The drawing under review shows one solid part. Ordinate dimensions are in mm from its lowest x, y, z. Round coordinates to 2 decimals unless told otherwise and drop trailing zeros. Write each loop counter-clockwise with the first axis right and the second up, starting at its lowest first coordinate (ties: lowest second). Pieces come first, ordered by that corner, then holes. Notation, with made-up numbers: (-15, 44) - (23, 44) arc R12 cw to (23, 60) - close; hole circle Ø11 at (-29.75, 42). An arc over 180 degrees is marked (long way). Answer in a Markdown table with one row per item. Add a question column.
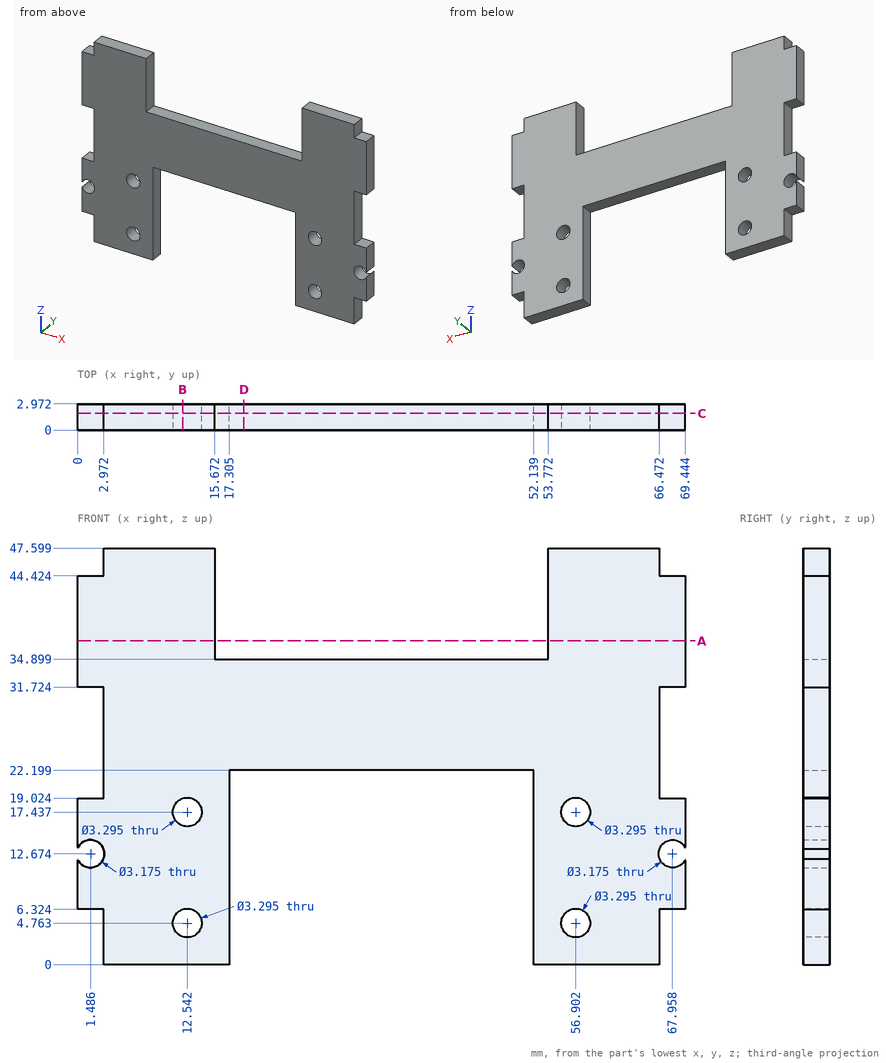
Q1. Add section A-A on z = 37. State the section outline as (x, y) points.
Q2. To check wall thickness, follow probe 1 along X at (y, z) = (2.55, 46); probe 2 along Z at (x, y) = (57, 2.55); probe 3 along Z at (x, y) = (56.5, 2) (1 decimal). State the ranges of each line that lie inside material, in increasing order.
Q3. Add section D-D on x = 19. State the section outline as (y, z) points.
Q4. Add section B-B on x = 12. State the section outline as (y, z) points, then the cut area to 3 significant figures.
Q5. Insertion check: pin 1 Ø0.9 at (x, y) = (67.5, 2) entering from +Z; pin 2 Ø0.9 at (x, y) = (1, 2) entering from -Z. Each pin has a flat end and moves straight along its axis. Give the tip position at first contact, or say it passes through.
Q6. Add section C-C on y = 1.9. Count the separate pieces of the cut face and the enclosed holes in it, then the cut area to 3 significant figures.
Answer sheet:
| question | item | result |
|---|---|---|
| 1 | outline | (0, 0) - (15.67, 0) - (15.67, 2.97) - (0, 2.97) - close; (53.77, 0) - (69.44, 0) - (69.44, 2.97) - (53.77, 2.97) - close |
| 2 | probe 1 | x = 2.97 to 15.67, 53.77 to 66.47 |
| 2 | probe 2 | z = 0 to 3.12, 6.41 to 15.79, 19.08 to 47.6 |
| 2 | probe 3 | z = 0 to 3.2, 6.4 to 15.8, 19 to 47.6 |
| 3 | outline | (0, 22.2) - (2.97, 22.2) - (2.97, 34.9) - (0, 34.9) - close |
| 4 | outline | (0, 0) - (2.97, 0) - (2.97, 3.21) - (0, 3.21) - close; (0, 6.32) - (2.97, 6.32) - (2.97, 15.88) - (0, 15.88) - close; (0, 18.99) - (2.97, 18.99) - (2.97, 47.6) - (0, 47.6) - close |
| 4 | area | 123 mm² |
| 5 | pin 1 | stops at z = 44.42 |
| 5 | pin 2 | stops at z = 6.32 |
| 6 | separate pieces | 1 |
| 6 | enclosed holes | 4 |
| 6 | area | 1,870 mm² |
